Here's how the part is built. I have some questions about the finished solid (model axes, mm). A direction names the side the tool comes from. Coordinates: 2 decimals unless noted, no trailing zeros. Loops run counter-clockwise (first coordinate to the right, second up) from the corner with the lowest first, then second, coordinate; pieces in that order, holes last. Notation, with made-up numbers: (88.5, 75.25) - (147.5, 75.25) arc R12 cw to (147.5, 95.25) - close; hole circle Ø5 at (59, -37.5). An arc over 180 degrees is marked (long way). Use a Markdown table: item, result.
```python
from build123d import *

# Parameters (mm, degrees)
SKETCH1_R                       = 3
SKETCH1_R_2                     = 13
SKETCH1_R_3                     = 2.5
BOSS_EXTRUDE1_DEPTH             = 2.5
CUT_EXTRUDE1_DEPTH              = 3.5
CUT_EXTRUDE1_DEPTH_BACK         = 3.5
BOSS_EXTRUDE2_REACH             = 4.5
BOSS_EXTRUDE2_DIRECTION_2_REACH = 4.5
FILLET2_R                       = 20
FILLET4_R                       = 6
FILLET5_R                       = 10
FILLET6_R                       = 3
FILLET7_R                       = 1.5


with BuildPart() as part:
    # Sketch1 → Boss-Extrude1 (new body, symmetric)
    with BuildSketch(Plane.XY):
        Polygon((-55, 10), (-110, 10), (-110, -10), (-55, -10), (-55, -55), (55, -55), (55, 55), (-55, 55), align=None)
        with Locations((0, 45)):
            Circle(SKETCH1_R, mode=Mode.SUBTRACT)
        with Locations((-44.598206242, -6)):
            Circle(SKETCH1_R, mode=Mode.SUBTRACT)
        with Locations((44.598206242, -6)):
            Circle(SKETCH1_R, mode=Mode.SUBTRACT)
        with Locations((11.3, -43.55812209)):
            Circle(SKETCH1_R, mode=Mode.SUBTRACT)
        Circle(SKETCH1_R_2, mode=Mode.SUBTRACT)
        with Locations((-95, 0)):
            Circle(SKETCH1_R_3, mode=Mode.SUBTRACT)
        with Locations((-70, 0)):
            Circle(SKETCH1_R_3, mode=Mode.SUBTRACT)
    extrude(amount=BOSS_EXTRUDE1_DEPTH, both=True)

    # Sketch2 → Cut-Extrude1 (cut, two sides)
    with BuildSketch(Plane.XY) as cut_extrude1_sk:
        Polygon((17.823700244, 55), (55, 12.487274774), (55, 55), align=None)
        Polygon((55, -24.415324997), (27.884298804, -55), (55, -55), align=None)
        Polygon((-7.739125069, -55), (-55, -24.068320295), (-55, -55), align=None)
        Polygon((-55, 55), (-18, 55), (-18, 39.905543875), (-35.675645396, 2), (-46.5, 2), (-46.5, 10), (-55, 10), align=None)
    extrude(amount=CUT_EXTRUDE1_DEPTH, mode=Mode.SUBTRACT)
    extrude(cut_extrude1_sk.sketch, amount=-CUT_EXTRUDE1_DEPTH_BACK, mode=Mode.SUBTRACT)

    # Boss-Extrude2: up to this face of the body (flat: up to its plane)
    boss_extrude2_end = Plane(part.part.faces().sort_by_distance((-48.483053202, 6, 2.5))[0])
    # Sketch3 → Boss-Extrude2 (add, up to the picked face)
    with BuildSketch(Plane.XY, mode=Mode.PRIVATE) as boss_extrude2_sk1:
        Polygon((-55, -24.068320295), (-76.495151, -10), (-55, -10), align=None)
    boss_extrude2_tool1 = split(extrude(boss_extrude2_sk1.sketch, amount=BOSS_EXTRUDE2_REACH, mode=Mode.PRIVATE), bisect_by=boss_extrude2_end, keep=Keep.BOTH, mode=Mode.PRIVATE)
    add(boss_extrude2_tool1.solids().sort_by_distance((-62.16505, -14.68944, 0))[0])

    # Boss-Extrude2 direction 2: up to this face of the body (flat: up to its plane)
    boss_extrude2_direction_2_end = Plane(part.part.faces().sort_by_distance((-78.25, 8.016946798, -2.5))[0])
    # Sketch3 → Boss-Extrude2 direction 2 (add, up to the picked face)
    with BuildSketch(Plane.XY, mode=Mode.PRIVATE) as boss_extrude2_direction_2_sk1:
        Polygon((-55, -24.068320295), (-76.495151, -10), (-55, -10), align=None)
    boss_extrude2_direction_2_tool1 = split(extrude(boss_extrude2_direction_2_sk1.sketch, amount=-BOSS_EXTRUDE2_DIRECTION_2_REACH, mode=Mode.PRIVATE), bisect_by=boss_extrude2_direction_2_end, keep=Keep.BOTH, mode=Mode.PRIVATE)
    add(boss_extrude2_direction_2_tool1.solids().sort_by_distance((-62.16505, -14.68944, 0))[0])

    # Fillet2
    fillet2_edges = [part.edges().sort_by_distance(p)[0] for p in [
        (-76.495151, -10, 0),
        (-7.739125069, -55, 0),
        (55, -24.415324997, 0),
        (27.884298804, -55, 0),
        (17.823700244, 55, 0),
        (55, 12.487274774, 0),
    ]]
    fillet(fillet2_edges, radius=FILLET2_R)

    # Fillet4
    fillet4_edges = [part.edges().sort_by_distance(p)[0] for p in [
        (-110, -10, 0),
        (-110, 10, 0),
    ]]
    fillet(fillet4_edges, radius=FILLET4_R)

    # Fillet5
    fillet5_edges = [part.edges().sort_by_distance(p)[0] for p in [
        (-18, 55, 0),
        (-18, 39.905543875, 0),
    ]]
    fillet(fillet5_edges, radius=FILLET5_R)

    # Fillet6
    fillet6_edges = [part.edges().sort_by_distance(p)[0] for p in [
        (-46.5, 10, 0),
    ]]
    fillet(fillet6_edges, radius=FILLET6_R)

    # Fillet7
    fillet7_edges = [part.edges().sort_by_distance(p)[0] for p in [
        (-35.675645396, 2, 0),
        (-46.5, 2, 0),
    ]]
    fillet(fillet7_edges, radius=FILLET7_R)


solid = part.part
```
Q1. I want a section at B-B, the plane x = -95. Write out the boundary of the cut face in (y, z), then the cut area to 3 significant figures.
Check values:
| item | result |
|---|---|
| outline | (-10, -2.5) - (-2.5, -2.5) - (-2.5, 2.5) - (-10, 2.5) - close; (2.5, -2.5) - (10, -2.5) - (10, 2.5) - (2.5, 2.5) - close |
| area | 75.0 mm^2 |
Q2. Please list where these lines run through material, in increasing order: L1, parallel to Y at x = 0, z = 1; L2, parallel to Y at x = -95, z = 1.35; L3, parallel to X at y = 8.5, z = 0. Write a range as from..to.
Check values:
| item | result |
|---|---|
| L1 | -55..-13, 13..42, 48..55 |
| L2 | -10..-2.5, 2.5..10 |
| L3 | -107.97..-46.9, -32.64..-9.84, 9.84..54.69 |
Q3. If we mould it in two halves opening along X, with no side actions, what happens to faces 1 (the face through (9.09, -41.53, -0.04)), 2 (the face through (-76, 10, 0)), 3 (the face through (42.022, -39.054, 0.035))? For each: pulls with the +X half, pulls with the -X half, needs draft (parallel to the pull), parting line crosses it, or undercut.
Check values:
| item | result |
|---|---|
| face 1 | undercut |
| face 2 | needs draft |
| face 3 | pulls with the +X half |
Q4. Will these pins go through, and if not, where does the flat tip stop? P1, Ø4, axis at x = -95, y = 0, coming from the +Z side; P2, Ø0.9, axis at y = 44, z = -1, coming from the -X side; P3, Ø3, axis at y = 34, z = 1.5, coming from the +X side.
Check values:
| item | result |
|---|---|
| P1 | through |
| P2 | x = -18 |
| P3 | x = 37.5 |
Q5. Which directions (+Z, -Z, +X, -X, +Y, -Y) give clear straight access to the entire face, cutting with the end or side of a thin tool? Please do faces 4 (the face through (36.744, 33.364, 0.035)), 5 (the face through (-26.99, 20.63, 0.04)).
Check values:
| item | result |
|---|---|
| face 4 | +Z, -Z, +X, +Y |
| face 5 | +Z, -Z, +Y |
Q6. I want a section at A-A, the plane x = 0. Write out the boundary of the cut face in (y, z), then the cut area to 3 significant figures.
Check values:
| item | result |
|---|---|
| outline | (-55, -2.5) - (-13, -2.5) - (-13, 2.5) - (-55, 2.5) - close; (13, -2.5) - (42, -2.5) - (42, 2.5) - (13, 2.5) - close; (48, -2.5) - (55, -2.5) - (55, 2.5) - (48, 2.5) - close |
| area | 390 mm^2 |
Q7. I want a section at D-D, the plane z = 1.4. Give the number of separate pieces and of enclosed holes in the cut face, then the cut area to 3 significant figures.
Check values:
| item | result |
|---|---|
| separate pieces | 1 |
| enclosed holes | 7 |
| area | 9,100 mm^2 |
Q8. I want a section at C-C, the plane y = 0. Write out the boundary of the cut face in (x, z).
Check values:
| item | result |
|---|---|
| outline | (-110, -2.5) - (-97.5, -2.5) - (-97.5, 2.5) - (-110, 2.5) - close; (-92.5, -2.5) - (-72.5, -2.5) - (-72.5, 2.5) - (-92.5, 2.5) - close; (-67.5, -2.5) - (-13, -2.5) - (-13, 2.5) - (-67.5, 2.5) - close; (13, -2.5) - (55, -2.5) - (55, 2.5) - (13, 2.5) - close |
